Autodesk Inventor part; units mm, degrees
ref_plane "YZ Plane" through (0, 0, 0) normal (1, 0, 0) x (0, 1, 0)
ref_plane "XZ Plane" through (0, 0, 0) normal (0, 1, 0) x (-1, 0, 0)
ref_plane "XY Plane" through (0, 0, 0) normal (0, 0, 1) x (1, 0, 0)
sketch "Sketch1" plane through (0, 0, 0) normal (0, 1, 0) x (-1, 0, 0)
  line L0 (0, 0) -> (40, 0)
  line L1 (40, 0) -> (40, -60)
  line L2 (40, -60) -> (0, -60)
  line L3 (0, -60) -> (0, 0)
  dimension "d0" = 40
  dimension "d1" = 60
extrude "Extrusion1" add sketch "Sketch1" along normal blind 7
sketch "Sketch2" plane through (0, 7, 0) normal (0, 1, 0) x (1, 0, 0)
  line L0 (-40, 0) -> (0, 0)
  line L1 (0, 0) -> (-24.276, 0)
  line L2 (-24.276, 0) -> (-24.276, 30)
  line L3 (-24.276, 30) -> (0, 30)
  line L4 (0, 30) -> (0, 0)
  dimension "d4" = 24.276
  dimension "d5" = 30
extrude "Extrusion2" cut sketch "Sketch2" against normal through all
sketch "Sketch3" plane through (0, 7, 0) normal (0, 1, 0) x (1, 0, 0)
  circle A0 centre (-20, 45) radius 6.4
  point P0 (0, 0)
  dimension "d8" = 12.8
extrude "Extrusion3" cut sketch "Sketch3" against normal blind 2.25
sketch "Sketch4" plane through (-20, 4.75, -45) normal (0, 1, 0) x (1, 0, 0)
  line L0 (-1.55, -1.55) -> (1.55, -1.55)
  line L1 (1.55, -1.55) -> (1.55, 1.55)
  line L2 (1.55, 1.55) -> (-1.55, 1.55)
  line L3 (-1.55, 1.55) -> (-1.55, -1.55)
  line L4 (-1.55, -1.55) -> (1.55, 1.55) construction
  line L5 (1.55, -1.55) -> (-1.55, 1.55) construction
  point P0 (20, -45)
  point P1 (0, 0)
  dimension "d11" = 3.1
  dimension "d12" = 3.1
extrude "Extrusion4" cut sketch "Sketch4" against normal blind 3
sketch "Sketch6" plane through (-18.45, 4.75, -43.45) normal (0, 0, -1) x (-1, 0, 0)
  circle A0 centre (1.5, -1.5) radius 1.5
  point P0 (-18.45, -4.75)
  dimension "d18" = 3
extrude "Extrusion6" cut sketch "Sketch6" against normal through all
sketch "Sketch7" plane through (0, 7, 0) normal (0, 1, 0) x (1, 0, 0)
  line L0 (-25.276, 17.3) -> (-21.276, 17.3)
  line L1 (-21.276, 17.3) -> (-21.276, 13.45)
  line L2 (-21.276, 13.45) -> (-25.276, 13.45)
  line L3 (-25.276, 13.45) -> (-25.276, 17.3)
  line L4 (-24.276, 0) -> (-24.276, 30)
  line L5 (-24.276, 30) -> (0, 30)
  point P0 (0, 0)
  dimension "d21" = 3.85
  dimension "d22" = 1
  dimension "d23" = 4
  dimension "d24" = 12.7
extrude "Extrusion7" cut sketch "Sketch7" against normal through all
properties part number "torch_light_injection_3d_pirnt_v0-1_20feb25" material "ABS Plastic"
Read the model definition and answer for the solid it produces. Units are mm, in the model's axes. A direction names the side the tool comes from. Give positions to 0.01 mm unless a question says otherwise; leave off trailing zeros. Loops run counter-clockwise (first coordinate to the right, second up) from the corner with the lowest first, then second, coordinate; pieces in that order, holes last. Notation, with made-up numbers: (57, -31.75) -> (73, -31.75) arc R31 cw to (73, 2.25) -> close; hole circle Ø11 at (-30, 81). An arc over 180 degrees is marked (long way). Use a Markdown table: item, result.
Q1. Section C-C, the plane y = 4 is taken. Determine the outline of the cut face in (x, z).
Solved:
| item | result |
|---|---|
| outline | (-40, -60) -> (0, -60) -> (0, -30) -> (-18.65, -30) -> (-18.65, -43.45) -> (-18.45, -43.45) -> (-18.45, -46.55) -> (-21.55, -46.55) -> (-21.55, -43.45) -> (-21.25, -43.45) -> (-21.25, -30) -> (-24.28, -30) -> (-24.28, -17.3) -> (-25.28, -17.3) -> (-25.28, -13.45) -> (-24.28, -13.45) -> (-24.28, 0) -> (-40, 0) -> close |
Q2. Section B-B, the plane z = -45 is taken. Determine the outline of the cut face in (x, y).
Solved:
| item | result |
|---|---|
| outline | (-40, 0) -> (0, 0) -> (0, 7) -> (-13.6, 7) -> (-13.6, 4.75) -> (-18.45, 4.75) -> (-18.45, 1.75) -> (-21.55, 1.75) -> (-21.55, 4.75) -> (-26.4, 4.75) -> (-26.4, 7) -> (-40, 7) -> close |
Q3. Determine the mould class of faces 6 (the face through (-20, 3, -60)), 7 (the face through (-20, 1.75, -45)), 8 (the face through (0, 3, -45)) for opening direction X: pulls with the +X half, pulls with the -X half, needs draft (parallel to the pull), parting line crosses it, or undercut.
Solved:
| item | result |
|---|---|
| face 6 | needs draft |
| face 7 | undercut |
| face 8 | pulls with the +X half |
Q4. Each of these flat-tipped pins is pushed along its axis until it touches: pin 1 (10 mm diameter, centred on x = -23, z = -47.5, fed in from +Y); pin 2 (2.5 mm diameter, centred on x = -20.5, z = -44.5, fed in from +Y); pin 3 (2 mm diameter, centred on x = -16, y = 3, fed in from +Z); pin 4 (3 mm diameter, centred on y = 3.5, z = -16, fed in from +X). Where does it stop, or does it pass through?
Solved:
| item | result |
|---|---|
| pin 1 | stops at y = 7 |
| pin 2 | stops at y = 4.75 |
| pin 3 | stops at z = -30 |
| pin 4 | stops at x = -24.28 |
Q5. A tool of negligible diameter and unlimited length cuts with its end or side. For faces 1 (the face through (-25.276, 4, -15)), 2 (the face through (-32, 3, 0)), 3 (the face through (-21.55, 3, -45)), 4 (the face through (-19.625, 1.786, -36.819)), 5 (the face through (-24.276, 4, -24)), from which of +Z, -Z, +X, -X, +Y, -Y can it reach the whole face along a straight path? Write none if from no direction.
Solved:
| item | result |
|---|---|
| face 1 | +X, +Y, -Y |
| face 2 | +Z, +X, -X, +Y, -Y |
| face 3 | +Y |
| face 4 | +Z |
| face 5 | +Z, +X, +Y, -Y |
Q6. Find the intervals of material crossed by line 1 along X through (y, z) = (3.25, -38); line 2 along X through (y, z) = (6.4, -45); line 3 along Y through (x, z) = (-19.95, -36.25), in increasing order.
Solved:
| item | result |
|---|---|
| line 1 | x = -40 to -21.45, -18.45 to 0 |
| line 2 | x = -40 to -26.4, -13.6 to 0 |
| line 3 | y = 0 to 1.75, 4.75 to 7 |
Q7. Section A-A, the plane z = -36 is taken. Determine the outline of the cut face in (x, y).
Solved:
| item | result |
|---|---|
| outline | (-40, 0) -> (0, 0) -> (0, 7) -> (-40, 7) -> close; hole circle Ø3 at (-19.95, 3.25) |
Q8. Section D-D, the plane x = -13 is taken. Determine the outline of the cut face in (y, z).
Solved:
| item | result |
|---|---|
| outline | (0, -60) -> (7, -60) -> (7, -30) -> (0, -30) -> close |
